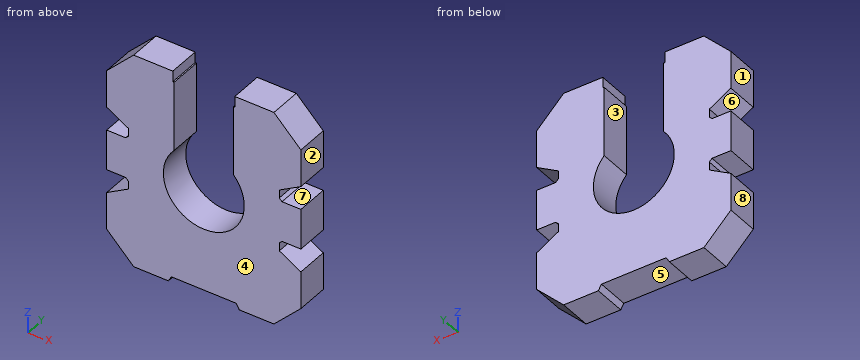
from build123d import *

# Parameters (mm, degrees)
SKETCH_1_W          = 360
SKETCH_1_H          = 400
EXTRUDE_1_DEPTH     = 60
CHAMFER_1_SIZE      = 50
SKETCH_2_W          = 40
SKETCH_2_H          = 115
CUT_EXTRUDE_1_DEPTH = 276.680975042
CUT_EXTRUDE_2_DEPTH = 60
SKETCH_4_W          = 110
SKETCH_4_H          = 95
SKETCH_4_H_2        = 20
SKETCH_4_W_2        = 2.5
CUT_EXTRUDE_3_DEPTH = 276.680975042
SKETCH_5_W          = 40
SKETCH_5_H          = 75
EXTRUDE_2_DEPTH     = 60
CUT_EXTRUDE_4_DEPTH = 60
SKETCH_7_R          = 75
CUT_EXTRUDE_5_DEPTH = 60
CUT_EXTRUDE_6_DEPTH = 60
CHAMFER_2_SIZE      = 5


with BuildPart() as part:
    # 草图1 → 凸台-拉伸1 (new body)
    with BuildSketch(Plane(origin=(0, 0, 0), x_dir=(1, 0, 0), z_dir=(0, 1, 0))):
        Rectangle(SKETCH_1_W, SKETCH_1_H)
    extrude(amount=EXTRUDE_1_DEPTH)

    # 倒角1
    chamfer_1_edges = [part.edges().sort_by_distance(p)[0] for p in [
        (180, 30, 200),
        (-180, 30, 200),
        (-180, 30, -200),
        (180, 30, -200),
    ]]
    chamfer(chamfer_1_edges, length=CHAMFER_1_SIZE)

    # 草图2 → 切除-拉伸1 (cut, through all)
    with BuildSketch(Plane(origin=(0, 60, 0), x_dir=(1, 0, 0), z_dir=(0, 1, 0))):
        with Locations((-160, 0)):
            Rectangle(SKETCH_2_W, SKETCH_2_H)
        with Locations((160, 0)):
            Rectangle(SKETCH_2_W, SKETCH_2_H)
    extrude(amount=-CUT_EXTRUDE_1_DEPTH, mode=Mode.SUBTRACT)

    # 草图3 → 切除-拉伸2 (cut)
    with BuildSketch(Plane(origin=(0, 60, 0), x_dir=(1, 0, 0), z_dir=(0, 1, 0))):
        Polygon((-140, -57.5), (-180, -57.5), (-180, -80.594010768), align=None)
        Polygon((-180, 80.594010768), (-140, 57.5), (-180, 57.5), align=None)
        Polygon((140, 57.5), (180, 57.5), (180, 80.594010768), align=None)
        Polygon((180, -80.594010768), (140, -57.5), (180, -57.5), align=None)
    extrude(amount=-CUT_EXTRUDE_2_DEPTH, mode=Mode.SUBTRACT)

    # 草图4 → 切除-拉伸3 (cut, through all)
    with BuildSketch(Plane(origin=(0, 0, 0), x_dir=(1, 0, 0), z_dir=(0, 1, 0))):
        with Locations((0, -132.5)):
            Rectangle(SKETCH_4_W, SKETCH_4_H)
        with Locations((0, -190)):
            Rectangle(SKETCH_4_W, SKETCH_4_H_2)
        with Locations((-56.25, -190)):
            Rectangle(SKETCH_4_W_2, SKETCH_4_H_2)
        with Locations((56.25, -190)):
            Rectangle(SKETCH_4_W_2, SKETCH_4_H_2)
    extrude(amount=CUT_EXTRUDE_3_DEPTH, mode=Mode.SUBTRACT)

    # 草图5 → 凸台-拉伸2 (add)
    with BuildSketch(Plane(origin=(0, 60, 0), x_dir=(1, 0, 0), z_dir=(0, 1, 0))):
        with Locations((-160, 0)):
            Rectangle(SKETCH_5_W, SKETCH_5_H)
        with Locations((160, 0)):
            Rectangle(SKETCH_5_W, SKETCH_5_H)
    extrude(amount=-EXTRUDE_2_DEPTH)

    # 草图6 → 切除-拉伸4 (cut)
    with BuildSketch(Plane(origin=(0, 60, 0), x_dir=(1, 0, 0), z_dir=(0, 1, 0))):
        Polygon((-65.773502692, 200), (-60, 190), (60, 190), (65.773502692, 200), align=None)
    extrude(amount=-CUT_EXTRUDE_4_DEPTH, mode=Mode.SUBTRACT)

    # 草图7 → 切除-拉伸5 (cut)
    with BuildSketch(Plane(origin=(0, 60, 0), x_dir=(1, 0, 0), z_dir=(0, 1, 0))):
        with Locations(Location((0, 0, 0), (0, 0, 270))):
            Circle(SKETCH_7_R)
    extrude(amount=-CUT_EXTRUDE_5_DEPTH, mode=Mode.SUBTRACT)

    # 草图8 → 切除-拉伸6 (cut)
    with BuildSketch(Plane(origin=(0, 60, 0), x_dir=(1, 0, 0), z_dir=(0, 1, 0))):
        with BuildLine():
            Line((-55, -85), (-55, -50.990195136))
            ThreePointArc((-55, -50.990195136), (0, -75), (55, -50.990195136))
            Line((55, -50.990195136), (55, -85))
            Line((55, -85), (-55, -85))
        make_face()
    extrude(amount=-CUT_EXTRUDE_6_DEPTH, mode=Mode.SUBTRACT)

    # 倒角2
    chamfer_2_edges = [part.edges().sort_by_distance(p)[0] for p in [
        (-140, 30, -37.5),
        (-140, 30, 37.5),
        (140, 30, 37.5),
        (140, 30, -37.5),
    ]]
    chamfer(chamfer_2_edges, length=CHAMFER_2_SIZE)


solid = part.part
Input: part model. Units: mm. Frame: model coordinates. Face numbers are marked on the shaded views. A direction names the side the tool comes from. Coordinates: 2 decimals unless noted, no trailing zeros. Loops run counter-clockwise (first coordinate to the right, second up) from the corner with the lowest first, then second, coordinate; pieces in that order, holes last. Notation, with made-up numbers: (11.25, -27.75) -> (48.25, -27.75) arc R19 ccw to (48.25, -18.75) -> close; hole circle Ø2 at (-31.75, 16). An arc over 180 degrees is marked (long way). Write item = value, one per line. Start each with the question number.
Item 1: First-contact query: P1, Ø0.8, axis at x = 55.5, y = 25, coming from the +Z side; P2, Ø4.5, axis at y = 27.5, z = -51, coming from the -X side; P3, Ø6, axis at x = -32, y = 8, coming from the +Z side; P4, Ø3, axis at x = -56.5, y = 32.5, coming from the +Z side. Flat tips, straight axial feed; report the tip coordinate or a pass-through.
Item 2: Cut plane D-D, the plane x = 36.5. Return loops of the section in (y, z), plus the area to 3 significant figures.
Item 3: Cut plane A-A, the plane z = 0. Return loops of the section in (x, y).
Item 4: Cut plane C-C, the plane z = 62. Return loops of the section in (x, y), plus the area to 3 significant figures.
Item 5: Material intervals for line 1 (X direction, y = 43, z = 0); line 2 (X direction, y = 21, z = 115.5); line 3 (Z direction, x = 0, y = 45), sorted ascending.
Item 6: Mould query, pull axis X, two halves, no side actions, for the marked faces 1, 2, 3 and 4. Classes: pulls with the +X half, pulls with the -X half, needs draft (parallel to the pull), parting line crosses it, or undercut.
Item 7: Reachability of the marked faces 5, 6, 7 and 8 from +Z, -Z, +X, -X, +Y, -Y: full face, straight path, thin tool, end or side. Return the list, or none.
Item 8: Cut plane B-B, the plane x = 0. Return loops of the section in (y, z).
Ans:
q1.P1 = 180
q1.P2 = -140
q1.P3 = -66.33
q1.P4 = 200
q2.outline = (0, -190) -> (60, -190) -> (60, -65.52) -> (0, -65.52) -> close
q2.area = 7,470 mm²
q3.outline = (-180, 0) -> (-75, 0) -> (-75, 60) -> (-180, 60) -> close; (75, 0) -> (180, 0) -> (180, 60) -> (75, 60) -> close
q4.outline = (-147.79, 0) -> (-55, 0) -> (-55, 60) -> (-147.79, 60) -> close; (55, 0) -> (147.79, 0) -> (147.79, 60) -> (55, 60) -> close
q4.area = 11,100 mm²
q5.line_1 = -180 to -75, 75 to 180
q5.line_2 = -180 to -55, 55 to 180
q5.line_3 = -190 to -75
q6.face_1 = pulls with the -X half
q6.face_2 = pulls with the +X half
q6.face_3 = undercut
q6.face_4 = needs draft
q7.face_5 = -Z, +Y, -Y
q7.face_6 = -X, +Y, -Y
q7.face_7 = +X, +Y, -Y
q7.face_8 = +Z, -Z, -X, +Y, -Y
q8.outline = (0, -190) -> (60, -190) -> (60, -75) -> (0, -75) -> close
